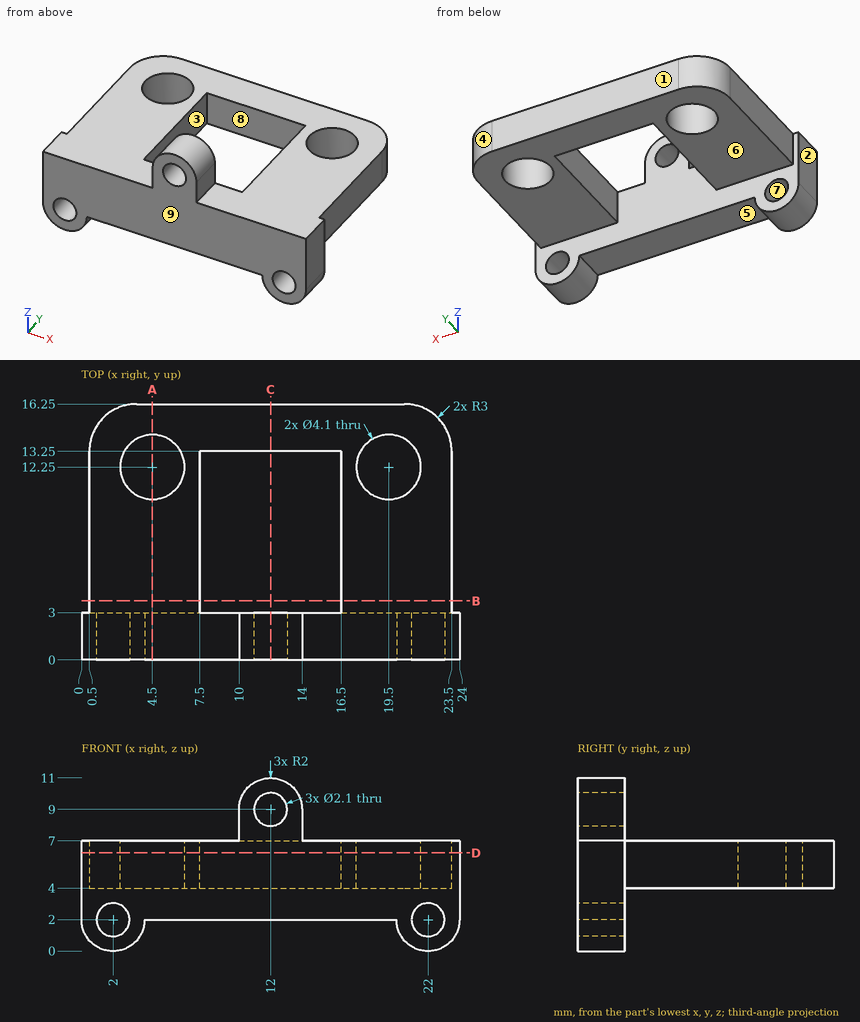
Job drawing, mm, ordinate dimensions from the low corner. One solid piece. A direction names the side the tool comes from. Round coordinates to 2 decimals unless told otherwise and drop trailing zeros. Order: outer loops, then holes, each group sorted by start corner. A loop starts at its lowest first (then second) coordinate and runs counter-clockwise, first axis right, second up. Notation, with made-up numbers: (-30.75, 38.5) -> (-6.75, 38.5) arc R19 ccw to (-6.75, 69.5) -> close; hole circle Ø8 at (85, -36.5). An arc over 180 degrees is marked (long way). Answer in a Markdown table with one row per item.
1) Mould opens along X. For the marked faces 1, 2, 3 and 4 say: released by +X, released by -X, zero draft, split by the parting line, or undercut.
Values:
| item | result |
|---|---|
| face 1 | zero draft |
| face 2 | released by -X |
| face 3 | undercut |
| face 4 | released by +X |
2) Pin check, flat tips, straight feed: P1, Ø5.5, axis at x = 19.5, y = 12.25, coming from the +Z side; P2, Ø2.5, axis at x = 22, z = 2, coming from the +Y side; P3, Ø3.5, axis at x = 13.5, z = 5.5, coming from the -Y side; P4, Ø1.9, axis at x = 2, z = 2, coming from the -Y side. Stop position of each tip, or through.
Values:
| item | result |
|---|---|
| P1 | z = 7 |
| P2 | y = 3 |
| P3 | y = 0 |
| P4 | through |
3) Wall check: L1, parallel to Z at x = 12, y = 0.85; L2, parallel to Z at x = 22, y = 1; L3, parallel to Y at x = 9, z = 6. Give the ranges that are in metal, low to high.
Values:
| item | result |
|---|---|
| L1 | 2 to 7.95, 10.05 to 11 |
| L2 | 0 to 0.95, 3.05 to 7 |
| L3 | 0 to 3, 13.25 to 16.25 |
4) Band-saw the part on B-B on y = 3.75. Give the cut face in (x, z).
Values:
| item | result |
|---|---|
| outline | (0.5, 4) -> (7.5, 4) -> (7.5, 7) -> (0.5, 7) -> close; (16.5, 4) -> (23.5, 4) -> (23.5, 7) -> (16.5, 7) -> close |
5) Which spindle directions (+Z, -Z, +X, -X, +Y, -Y) get a long thin tool onto all of the face, cutting with end or side? Do the marked faces 5, 6, 7, 8 and 9. Say none if no direction does.
Values:
| item | result |
|---|---|
| face 5 | -Z, +Y, -Y |
| face 6 | -Z, +X, -X, +Y |
| face 7 | +Y, -Y |
| face 8 | +Z, -Z |
| face 9 | +Z, -Z, +X, -X, -Y |
6) Band-saw the part on D-D on z = 6.25. Give the cut face in (x, y).
Values:
| item | result |
|---|---|
| outline | (0, 0) -> (24, 0) -> (24, 3) -> (23.5, 3) -> (23.5, 13.25) arc R3 ccw to (20.5, 16.25) -> (3.5, 16.25) arc R3 ccw to (0.5, 13.25) -> (0.5, 3) -> (0, 3) -> close; hole circle Ø4.1 at (4.5, 12.25); hole (7.5, 3) -> (16.5, 3) -> (16.5, 13.25) -> (7.5, 13.25) -> close; hole circle Ø4.1 at (19.5, 12.25) |
7) Band-saw the part on C-C on x = 12. Give the cut face in (y, z), and give its area (3 significant figures).
Values:
| item | result |
|---|---|
| outline | (0, 2) -> (3, 2) -> (3, 7.95) -> (0, 7.95) -> close; (0, 10.05) -> (3, 10.05) -> (3, 11) -> (0, 11) -> close; (13.25, 4) -> (16.25, 4) -> (16.25, 7) -> (13.25, 7) -> close |
| area | 29.7 mm2 |
8) Band-saw the part on A-A on x = 4.5. Give the cut face in (y, z), and give its area (4 significant figures).
Values:
| item | result |
|---|---|
| outline | (0, 2) -> (3, 2) -> (3, 4) -> (10.2, 4) -> (10.2, 7) -> (0, 7) -> close; (14.3, 4) -> (16.25, 4) -> (16.25, 7) -> (14.3, 7) -> close |
| area | 42.45 mm2 |
